Geometry: final body of the model. Coordinates: model frame, mm. Face numbers are marked on the shaded views. A direction names the side the tool comes from. Round coordinates to 2 decimals unless told otherwise and drop trailing zeros. Loops run counter-clockwise (first coordinate to the right, second up) from the corner with the lowest first, then second, coordinate; pieces in that order, holes last. Notation, with made-up numbers: (-36.5, -8) - (15.5, -8) arc R16 ccw to (15.5, 6) - close; hole circle Ø2 at (5, 18.5). An arc over 180 degrees is marked (long way). Answer as CSV lines item,"result".
from build123d import *

# Parameters (mm, degrees)
F1_DEPTH = 100


with BuildPart() as f1:
    # F0 (on Front) → F1 (new body)
    with BuildSketch(Plane.XZ):
        with BuildLine():
            ThreePointArc((-20, 0), (-15.320889, 12.855752), (-3.472964, 19.696155))
            Line((-3.472964, 19.696155), (-3.82026, 21.665771))
            ThreePointArc((-3.82026, 21.665771), (-16.852978, 14.141327), (-22, 0))
            Line((-22, 0), (-22, -21.897534))
            Line((-22, -21.897534), (-20, -21.897534))
            Line((-20, -21.897534), (-20, 0))
        make_face()
    extrude(amount=F1_DEPTH)


solid = f1.part
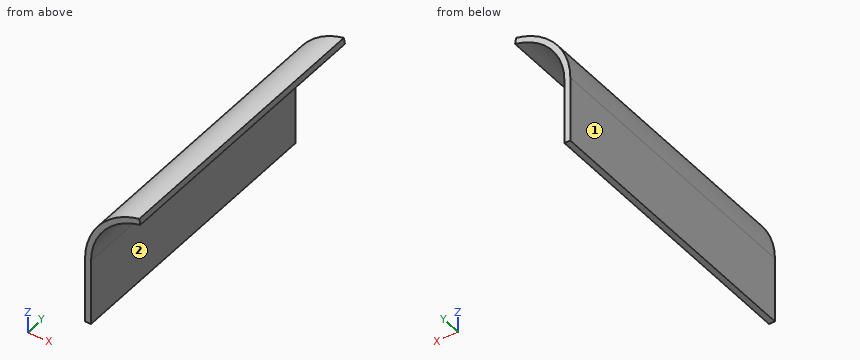
(1) Access query for the marked faces 1 and 2. Directions: +Z, -Z, +X, -X, +Y, -Y. A direction counts if a zero-diameter tool reaches every point of the face in a straight line with its end or side. Return the directions, or none.
Findings below:
face 1,"+Z, -Z, -X, +Y, -Y"
face 2,"-Z, +X, +Y, -Y"
(2) Section A-A (z = -4). Output: boundary loops of the cut face in (x, y).
Findings below:
outline,"(-22, -100) - (-20, -100) - (-20, 0) - (-22, 0) - close"
(3) Section C-C (x = -9.75). Output: boundary loops of the cut face in (y, z).
Findings below:
outline,"(-100, 17.46) - (0, 17.46) - (0, 19.72) - (-100, 19.72) - close"
(4) Section B-B (y = -26.5). Output: boundary loops of the cut face in (x, z), and give its area (3 significant figures).
Findings below:
outline,"(-22, -21.9) - (-20, -21.9) - (-20, 0) arc R20 cw to (-3.47, 19.7) - (-3.82, 21.67) arc R22 ccw to (-22, 0) - close"
area,"102 mm2"
(5) Pin query (flat end, axial travel): P1, Ø4, axis at y = -88, z = -14, coming from the +X side; P2, Ø8, axis at x = -5.5, y = -20.5, coming from the +Z side; P3, Ø1.5, axis at x = -15, y = -64, coming from the -Z side; P4, Ø8, axis at x = -12.5, z = -7, coming from the -Y side. Return the tip coordinate at first contact, or that it passes through.
Findings below:
P1,"x = -20"
P2,"z = 21.67"
P3,"z = 12.33"
P4,"through"
(6) Material intervals for line 1 along X through (y, z) = (-49, -17); line 2 along Z through (x, y) = (-8.5, -27); line 3 along Z through (x, y) = (-13, -24.5), sorted ascending.
Findings below:
line 1,"-22 to -20"
line 2,"18.1 to 20.29"
line 3,"15.2 to 17.75"
